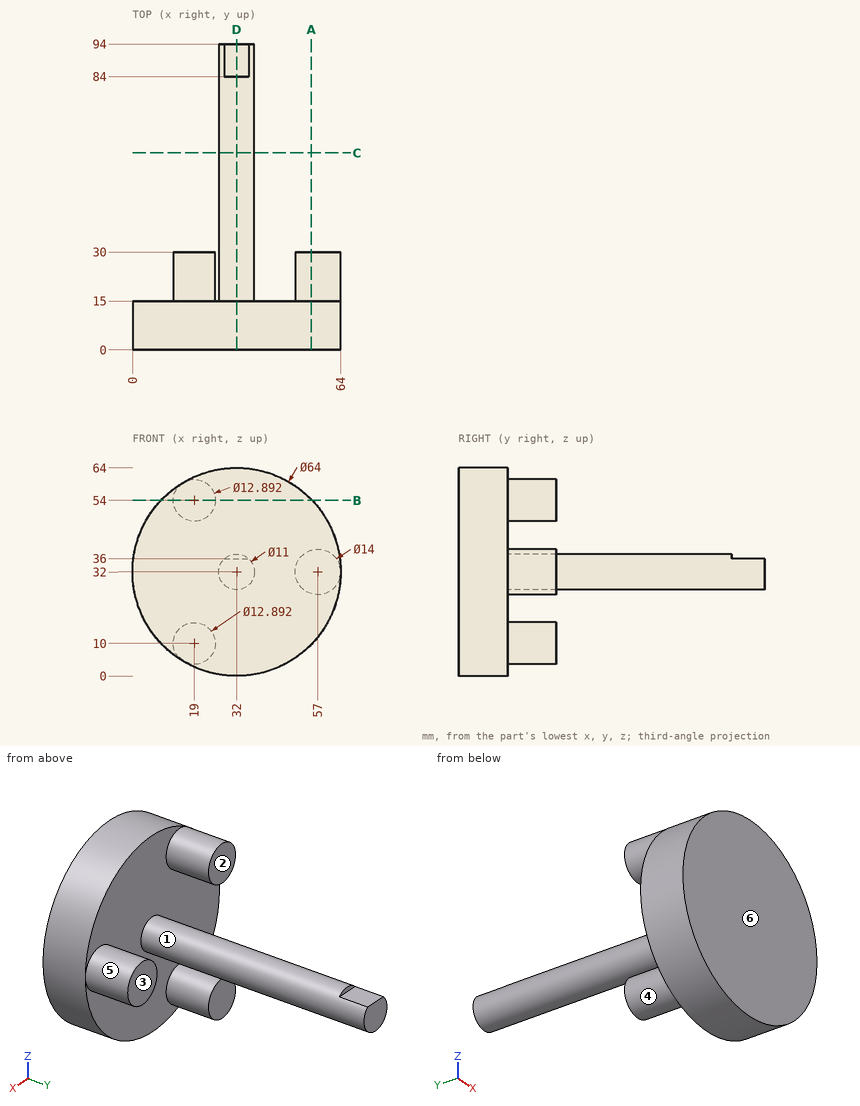
Geometry: see drawing. Coordinates: mm, zero at the bounding-box minimum. A direction names the side the tool comes from. Give positions to 0.01 mm unless a question says otherwise; leave off trailing zeros. Write each loop counter-clockwise with the first axis right and the second up, starting at its lowest first coordinate (ties: lowest second). Pieces come first, ordered by that corner, then holes. Notation, with made-up numbers: M -38.5,-20.75 L 11.5,-20.75 A18 ccw 11.5,-10.75 Z; hole C -9.5,76 d10. An arc over 180 degrees is marked long. Return JSON: item names as keys, results as strings. Group by question number.
1) Cut plane C-C, the plane y = 60.5. Output: boundary loops of the cut face in (x, z).
2) Cut plane B-B, the plane z = 54. Output: boundary loops of the cut face in (x, y).
3) Set-up query: the marked faces 1, 2 and 3. Return all of +Z, -Z, +X, -X, +Y, -Y with unobstructed straight access to the full face (end or side cutting, diameter ignored); none if empty.
4) Draft query along X for the marked faces 4, 5 and 6. Return one class per face: released by +X, released by -X, zero draft, split by the parting line, or undercut.
5) Ray query, L1, parallel to Y at x = 26, z = 44.5; L2, parallel to Z at x = 20, y = 24.5; L3, parallel to Z at x = 35, y = 50. Return the intervals inside material, ascending.
6) Cut plane A-A, the plane x = 55. Output: boundary loops of the cut face in (y, z).
7) First-contact query: pin 1 Ø12 at (x, y) = (28, 70.5) entering from +Z; pin 2 Ø4 at (x, y) = (29, 17.5) entering from -Z; pin 3 Ø0.8 at (x, z) = (33.5, 37) entering from +Y. Flat tips, straight axial feed; report the tip coordinate or a pass-through.
8) Cut plane D-D, the plane x = 32. Output: boundary loops of the cut face in (y, z), then the cut area to 3 significant figures.
Data:
{
 "1": {"outline": "C 32,32 d11"},
 "2": {"outline": "M 8.76,0 L 55.24,0 L 55.24,15 L 25.45,15 L 25.45,30 L 12.55,30 L 12.55,15 L 8.76,15 Z"},
 "3": {"face 1": "+Y", "face 2": "+Z, -Z, +X, -X, +Y", "face 3": "+Z, -Z, +X, +Y"},
 "4": {"face 4": "split by the parting line", "face 5": "undercut", "face 6": "zero draft"},
 "5": {"L1": "y = 0 to 15", "L2": "z = 3.63 to 16.37, 47.63 to 60.37", "L3": "z = 27.39 to 36.61"},
 "6": {"outline": "M 0,9.75 L 15,9.75 L 15,25.29 L 30,25.29 L 30,38.71 L 15,38.71 L 15,54.25 L 0,54.25 Z"},
 "7": {"pin 1": "stops at z = 37.5", "pin 2": "stops at z = 26.59", "pin 3": "stops at y = 84"},
 "8": {"outline": "M 0,0 L 15,0 L 15,26.5 L 94,26.5 L 94,36 L 84,36 L 84,37.5 L 15,37.5 L 15,64 L 0,64 Z", "area": "1,810 mm²"}
}
